```python
from build123d import *

# Parameters (mm, degrees)
SKETCH1_R                = 21
SKETCH1_R_2              = 13.5
BOSS_EXTRUDE1_DEPTH      = 5
BOSS_EXTRUDE2_REACH      = 49.223
BOSS_EXTRUDE2_END_RADIUS = 21
SKETCH2_W                = 5
SKETCH2_H                = 42
SKETCH2_3_W              = 45
SKETCH2_3_H              = 42
SKETCH2_3_R              = 3
BOSS_EXTRUDE3_DEPTH      = 5
CUT_EXTRUDE4_DEPTH       = 62.684682053


with BuildPart() as part:
    # Sketch1 → Boss-Extrude1 (new body)
    with BuildSketch(Plane(origin=(0, 0, 0), x_dir=(0, 0, -1), z_dir=(1, 0, 0))):
        Circle(SKETCH1_R)
        Circle(SKETCH1_R_2, mode=Mode.SUBTRACT)
    extrude(amount=BOSS_EXTRUDE1_DEPTH)

    # Boss-Extrude2: up to this cylinder (the profile starts outside it)
    boss_extrude2_end = Plane(origin=(2.5, 0, 0), z_dir=(-1, 0, 0)) * Cylinder(BOSS_EXTRUDE2_END_RADIUS, 141.446, mode=Mode.PRIVATE)
    # Sketch2 → Boss-Extrude2 (add, up to the surface)
    with BuildSketch(Plane(origin=(0, 21, 0), x_dir=(1, 0, 0), z_dir=(0, 1, 0)), mode=Mode.PRIVATE) as boss_extrude2_sk1:
        with Locations((2.5, 0)):
            Rectangle(SKETCH2_W, SKETCH2_H)
    boss_extrude2_tool1 = extrude(boss_extrude2_sk1.sketch, amount=-BOSS_EXTRUDE2_REACH, mode=Mode.PRIVATE) - boss_extrude2_end
    add(boss_extrude2_tool1.solids().sort_by_distance((2.5, 21, 0))[0])
    add(boss_extrude2_tool1.solids().sort_by_distance((2.5, 21, 0))[1])

    # Sketch2_3 → Boss-Extrude3 (add)
    with BuildSketch(Plane(origin=(0, 21, 0), x_dir=(1, 0, 0), z_dir=(0, 1, 0))):
        with Locations((-17.5, 0)):
            Rectangle(SKETCH2_3_W, SKETCH2_3_H)
        with Locations(Location((-35, 0, 0), (0, 0, 270))):
            Circle(SKETCH2_3_R, mode=Mode.SUBTRACT)
    extrude(amount=BOSS_EXTRUDE3_DEPTH)

    # Sketch3 → Cut-Extrude4 (cut, through all)
    with BuildSketch(Plane.XZ.offset(-21)):
        Polygon((0, -28.471778575), (0, -21), (-40, -7.216009452), (-40, -28.471778575), align=None)
        Polygon((-40, 7.216009452), (0, 21), (0, 27.25128432), (-40, 27.25128432), align=None)
    extrude(amount=-CUT_EXTRUDE4_DEPTH, mode=Mode.SUBTRACT)


solid = part.part
```
Can you work these out from the model? Positions are in its coordinate system, mm. A direction names the side the tool comes from. Give positions to 0.01 mm unless a question says otherwise; leave off trailing zeros. Order: outer loops, then holes, each group sorted by start corner. A loop starts at its lowest first (then second) coordinate and runs counter-clockwise, first axis right, second up. Notation, with made-up numbers: (-35, 62.25) - (-9, 62.25) arc R14 ccw to (-9, 73.25) - close; hole circle Ø3 at (-38, 7.5). An arc over 180 degrees is marked (long way). Use a Markdown table: item, result. Add a question column.
Q1. If we section it at A-A on z = 0: Write out the boundary of the cut face in (x, y), plus the area to 3 significant figures.
Q2. I'm going to push flat-ended pins straight in: pin 1 (20 mm diameter, centred on x = -19.5, z = 4.5, fed in from -Y); pin 2 (21 mm diameter, centred on y = 8.5, z = -6, fed in from -X); pin 3 (5 mm diameter, centred on y = 20.5, z = 4.5, fed in from -X). Where does each tip first touch, or does it pass through?
Q3. If we section it at D-D on z = 11: Write out the boundary of the cut face in (x, y).
Q4. If we section it at C-C on x = -35: Write out the boundary of the cut face in (y, z), plus the area to 3 significant figures.
Q5. If we mould it in two halves opening along Y, with no side actions, what happens to faces 1 (the flat face through (-19.72, 23.465, -14.204)), 2 (the flat face through (-16, 21, 0)), 3 (the cylindrical face through (2.46, -13.18, 2.93))? For each: released by +Y, released by -Y, zero draft, split by the parting line, or undercut.
Q6. If we section it at B-B on y = 11: Write out the boundary of the cut face in (x, z), plus the area to 3 significant figures.
Q7. Please list where these lines run through material, in increasing order: line 1 along X through (y, z) = (23, 0); line 2 along Y through (x, z) = (2.45, 0); line 3 along Y through (x, z) = (-3, 13).
Q8. On a 3-axis mill with a long thin cutter (end or side, diameter ignored), from which of +Z, -Z, +X, -X, +Y, -Y can I reach the whole of each face in a straight line? I mean faces 4 (the flat face through (-40, 23, 0)), 5 (the flat face through (0, 14, 0)). Say none if no direction works.
Answers follow:
| question | item | result |
|---|---|---|
| 1 | outline | (-40, 21) - (-38, 21) - (-38, 26) - (-40, 26) - close; (-32, 21) - (0, 21) - (0, 13.5) - (5, 13.5) - (5, 26) - (-32, 26) - close; (0, -21) - (5, -21) - (5, -13.5) - (0, -13.5) - close |
| 1 | area | 270 mm^2 |
| 2 | pin 1 | stops at y = 21 |
| 2 | pin 2 | stops at x = 0 |
| 2 | pin 3 | stops at x = -40 |
| 3 | outline | (-29.02, 21) - (0, 21) - (0, 7.83) - (5, 7.83) - (5, 26) - (-29.02, 26) - close; (0, -17.89) - (5, -17.89) - (5, -7.83) - (0, -7.83) - close |
| 4 | outline | (21, -8.94) - (26, -8.94) - (26, -3) - (21, -3) - close; (21, 3) - (26, 3) - (26, 8.94) - (21, 8.94) - close |
| 4 | area | 59.4 mm^2 |
| 5 | face 1 | zero draft |
| 5 | face 2 | released by -Y |
| 5 | face 3 | undercut |
| 6 | outline | (0, -21) - (5, -21) - (5, -7.83) - (0, -7.83) - close; (0, 7.83) - (5, 7.83) - (5, 21) - (0, 21) - close |
| 6 | area | 132 mm^2 |
| 7 | line 1 | x = -40 to -38, -32 to 5 |
| 7 | line 2 | y = -21 to -13.5, 13.5 to 26 |
| 7 | line 3 | y = 21 to 26 |
| 8 | face 4 | +Z, -Z, -X, +Y, -Y |
| 8 | face 5 | +Z, -Z, -X, -Y |
